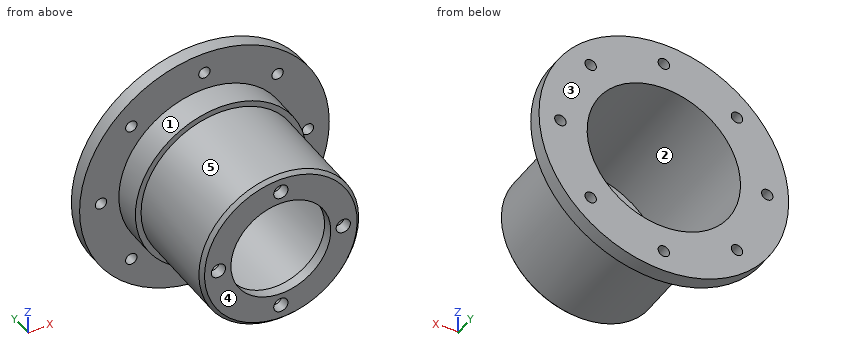
from build123d import *

# Parameters (mm, degrees)
SKETCH_1_R      = 22.4
SKETCH_1_R_2    = 14
SKETCH_1_R_3    = 2
EXTRUDE_1_DEPTH = 3
EXTRUDE_START   = 34
SKETCH_1_3_R    = 22.4
SKETCH_1_3_R_2  = 21.5
EXTRUDE_2_DEPTH = 34
EXTRUDE_START_2 = 4
SKETCH_2_R      = 35
SKETCH_2_R_2    = 21.5
SKETCH_2_R_3    = 1.6
EXTRUDE_3_DEPTH = 4
SKETCH_3_R      = 24
SKETCH_3_R_2    = 22.4
EXTRUDE_4_DEPTH = 8
CHAMFER_1_SIZE  = 1


with BuildPart() as part:
    # Sketch 1 → Extrude 1 (new body)
    with BuildSketch(Plane(origin=(0, 0, 0), x_dir=(1, 0, 0), z_dir=(0, 1, 0))):
        with Locations(Location((0, 0, 0), (0, 0, 270))):
            Circle(SKETCH_1_R)
        with Locations(Location((0, 0, 0), (0, 0, 270))):
            Circle(SKETCH_1_R_2, mode=Mode.SUBTRACT)
        with Locations(Location((17.5, 0, 0), (0, 0, 270))):
            Circle(SKETCH_1_R_3, mode=Mode.SUBTRACT)
        with Locations(Location((0, -17.5, 0), (0, 0, 270))):
            Circle(SKETCH_1_R_3, mode=Mode.SUBTRACT)
        with Locations(Location((-17.5, 0, 0), (0, 0, 270))):
            Circle(SKETCH_1_R_3, mode=Mode.SUBTRACT)
        with Locations(Location((0, 17.5, 0), (0, 0, 270))):
            Circle(SKETCH_1_R_3, mode=Mode.SUBTRACT)
    extrude(amount=-EXTRUDE_1_DEPTH)

    # Sketch 1_3 → Extrude 2 (add)
    with BuildSketch(Plane(origin=(0, 0, 0), x_dir=(1, 0, 0), z_dir=(0, 1, 0)).offset(EXTRUDE_START)):
        with Locations(Location((0, 0, 0), (0, 0, 270))):
            Circle(SKETCH_1_3_R)
        with Locations(Location((0, 0, 0), (0, 0, 270))):
            Circle(SKETCH_1_3_R_2, mode=Mode.SUBTRACT)
    extrude(amount=-EXTRUDE_2_DEPTH)

    # Sketch 2 → Extrude 3 (add)
    with BuildSketch(Plane(origin=(0, 34, 0), x_dir=(1, 0, 0), z_dir=(0, 1, 0)).offset(EXTRUDE_START_2)):
        with Locations(Location((0, 0, 0), (0, 0, 270))):
            Circle(SKETCH_2_R)
        with Locations(Location((0, 0, 0), (0, 0, 270))):
            Circle(SKETCH_2_R_2, mode=Mode.SUBTRACT)
        with Locations(Location((29, 0, 0), (0, 0, 270))):
            Circle(SKETCH_2_R_3, mode=Mode.SUBTRACT)
        with Locations(Location((20.506096654, -20.506096654, 0), (0, 0, 270))):
            Circle(SKETCH_2_R_3, mode=Mode.SUBTRACT)
        with Locations(Location((0, -29, 0), (0, 0, 270))):
            Circle(SKETCH_2_R_3, mode=Mode.SUBTRACT)
        with Locations(Location((-20.506096654, -20.506096654, 0), (0, 0, 270))):
            Circle(SKETCH_2_R_3, mode=Mode.SUBTRACT)
        with Locations(Location((-29, 0, 0), (0, 0, 270))):
            Circle(SKETCH_2_R_3, mode=Mode.SUBTRACT)
        with Locations(Location((-20.506096654, 20.506096654, 0), (0, 0, 270))):
            Circle(SKETCH_2_R_3, mode=Mode.SUBTRACT)
        with Locations(Location((0, 29, 0), (0, 0, 270))):
            Circle(SKETCH_2_R_3, mode=Mode.SUBTRACT)
        with Locations(Location((20.506096654, 20.506096654, 0), (0, 0, 270))):
            Circle(SKETCH_2_R_3, mode=Mode.SUBTRACT)
    extrude(amount=-EXTRUDE_3_DEPTH)

    # Sketch 3 → Extrude 4 (add)
    with BuildSketch(Plane.XZ.offset(-34)):
        with Locations(Location((0, 0, 0), (0, 0, 90))):
            Circle(SKETCH_3_R)
        with Locations(Location((0, 0, 0), (0, 0, 90))):
            Circle(SKETCH_3_R_2, mode=Mode.SUBTRACT)
    extrude(amount=EXTRUDE_4_DEPTH)

    # Chamfer 1
    chamfer_1_edges = [part.edges().sort_by_distance(p)[0] for p in [
        (0, -3, -22.4),
    ]]
    chamfer(chamfer_1_edges, length=CHAMFER_1_SIZE)


solid = part.part
Build history of the part. All positions in model axes, mm. Face numbers are marked on the shaded views. A direction names the side the tool comes from. Round coordinates to 2 decimals unless told otherwise and drop trailing zeros. Order: outer loops, then holes, each group sorted by start corner. A loop starts at its lowest first (then second) coordinate and runs counter-clockwise, first axis right, second up. Notation, with made-up numbers: M 78,66 L 115,66 A15 cw 115,80 Z; hole C -13.5,87 d9. An arc over 180 degrees is marked long. Use CSV: the item, a comma, the result in double quotes. Start each with the question number.
(1) Cut at C-C on x = 29. List the corners of the cut face in (y, z), then the cut area to 3 significant figures.
(2) Mould opens along Z. For the marked faces 1, 2 and 3 say: +Z half, -Z half, draft (parallel to the pull), parting line (faces both ways), or undercut.
(3) Cut at A-A on z = 29. List the corners of the cut face in (x, y), then the cut area to 3 significant figures.
(4) Drill centre lines: probe 1 along Z at (x, y) = (-0.5, 21.5); probe 2 along Y at (x, z) = (-11, -29); probe 3 along X at (y, z) = (35.9, 29). Where is each one in solid material? Low to high.
(5) Flat gauge pins, fed straight in: P1, Ø21.5, axis at x = -2.5, z = 9, coming from the +Y side; P2, Ø3, axis at x = 20.51, z = -20.51, coming from the -Y side; P3, Ø1.5, axis at x = 6, y = 13.5, coming from the +Z side; P4, Ø5, axis at x = 20.51, z = 20.51, coming from the -Y side. Where does each tip first touch, or does it go through?
(6) Tool access for the marked faces 4 and 5: list every direction of +Z, -Z, +X, -X, +Y, -Y with a clear straight run to the whole face (end or side of a thin tool).
(7) Cut at D-D on y = 12. List the corners of the cut face in (x, z), then the cut area to 3 significant figures.
(8) Cut at B-B on y = 35. State how many separate pieces and enclosed holes the cut face has, then the cut area to 3 significant figures.
Findings:
1,outline,"M 34,-19.6 L 38,-19.6 L 38,-1.6 L 34,-1.6 Z; M 34,1.6 L 38,1.6 L 38,19.6 L 34,19.6 Z"
1,area,"144 mm^2"
2,face 1,"parting line"
2,face 2,"undercut"
2,face 3,"draft"
3,outline,"M -19.6,34 L -1.6,34 L -1.6,38 L -19.6,38 Z; M 1.6,34 L 19.6,34 L 19.6,38 L 1.6,38 Z"
3,area,"144 mm^2"
4,probe 1,"z = -22.39 to -21.49, 21.49 to 22.39"
4,probe 2,"y = 34 to 38"
4,probe 3,"x = -19.6 to -1.6, 1.6 to 19.6"
5,P1,"stops at y = 0"
5,P2,"passes through"
5,P3,"stops at z = 21.78"
5,P4,"stops at y = 34"
6,face 4,"+Z, -Z, +X, -X, -Y"
6,face 5,"-Y"
7,outline,"C 0,0 d44.8; hole C 0,0 d43"
7,area,"124 mm^2"
8,separate pieces,"1"
8,enclosed holes,"9"
8,area,"2,330 mm^2"
